Could you check a few things on this model? Use its own coordinates, in mm. A direction names the side the tool comes from. Give positions to 0.01 mm unless a question says otherwise; leave off trailing zeros. Loops run counter-clockwise (first coordinate to the right, second up) from the corner with the lowest first, then second, coordinate; pieces in that order, holes last. Notation, with made-up numbers: (15, 41) -> (60, 41) arc R9 cw to (60, 48) -> close; hole circle Ø9 at (24, -36). An arc over 180 degrees is marked (long way). Put each result on its own line as item: value.
```python
from build123d import *

# Parameters (mm, degrees)
F0_R     = 14
F1_DEPTH = 3
F2_R     = 4
F3_DEPTH = 1.25
F5_DEPTH = 11.5
F6_DEPTH = 25.4
F4_R     = 1.75
F7_DEPTH = 25.4


# Not quite as in the source:
# - a feature names something its author has since deleted; it is built from what else it names


with BuildPart() as f1:
    # F0 (on Top) → F1 (new body)
    with BuildSketch(Plane.XY):
        with Locations((-41.5364727378, -7.5015998445)):
            Circle(F0_R)
    extrude(amount=F1_DEPTH)

    # F2 (on face) → F3 (cut)
    with BuildSketch(Plane.XY.offset(3)):
        with Locations((-41.5364727378, -7.5015998445)):
            Circle(F2_R)
    extrude(amount=-F3_DEPTH, mode=Mode.SUBTRACT)

    # F4 (on face) → F5 (join)
    with BuildSketch(Plane.XY.offset(3)):
        with BuildLine():
            ThreePointArc((-46.2922708097, -1.256661386), (-49.6170112359, -0.6113276981), (-46.7751178459, -2.4536079239))
            ThreePointArc((-46.7751178459, -2.4536079239), (-46.4175303835, -1.9019950739), (-46.2922708097, -1.256661386))
        make_face()
        with BuildLine():
            ThreePointArc((-33.3423393435, -13.758620951), (-34.4205133346, -12.1594833352), (-36.3072565774, -12.5593585722))
            ThreePointArc((-36.3072565774, -12.5593585722), (-35.7141653523, -15.3577585668), (-33.3423393435, -13.758620951))
        make_face()
        with BuildLine():
            ThreePointArc((-46.0564111963, -13.9823979165), (-46.193904066, -13.3075304398), (-46.5844646585, -12.7402449527))
            ThreePointArc((-46.5844646585, -12.7402449527), (-49.3689183267, -14.6572653931), (-46.0564111963, -13.9823979165))
        make_face()
        with BuildLine():
            ThreePointArc((-33.5665342792, -1.0208017726), (-35.9664017559, 0.5667053577), (-36.4884808171, -2.2629547364))
            ThreePointArc((-36.4884808171, -2.2629547364), (-34.6166668026, -2.608308903), (-33.5665342792, -1.0208017726))
        make_face()
    extrude(amount=-F5_DEPTH)

    # F4 (on face) → F6 (cut)
    with BuildSketch(Plane.XY.offset(3)):
        with BuildLine():
            ThreePointArc((-39.7864727378, 1.9984001555), (-42.7739096049, 3.2358370225), (-41.5364727378, 0.2484001555))
            ThreePointArc((-41.5364727378, 0.2484001555), (-40.2990358707, 0.7609632884), (-39.7864727378, 1.9984001555))
        make_face()
        with BuildLine():
            ThreePointArc((-31.2864727378, -7.5015998445), (-33.0364727378, -5.7515998445), (-34.7864727378, -7.5015998445))
            ThreePointArc((-34.7864727378, -7.5015998445), (-33.0364727378, -9.2515998445), (-31.2864727378, -7.5015998445))
        make_face()
        with BuildLine():
            ThreePointArc((-39.7864727378, -17.0011998445), (-40.2990358707, -15.7637629775), (-41.5364727378, -15.2511998445))
            ThreePointArc((-41.5364727378, -15.2511998445), (-42.7739096049, -18.2386367116), (-39.7864727378, -17.0011998445))
        make_face()
    extrude(amount=-F6_DEPTH, mode=Mode.SUBTRACT)

    # F4 (on face) → F7 (cut)
    with BuildSketch(Plane.XY.offset(3)):
        with Locations((-50.0454727378, -7.5015998445)):
            Circle(F4_R)
    extrude(amount=-F7_DEPTH, mode=Mode.SUBTRACT)


solid = f1.part
```
1. If we section it at B-B (x = -32.75): List the corners of the cut face in (y, z) for me, then the cut area to 3 significant figures.
Recorded:
outline: (-18.4, 0) -> (-9.23, 0) -> (-9.23, 3) -> (-18.4, 3) -> close; (-5.78, 0) -> (3.4, 0) -> (3.4, 3) -> (-5.78, 3) -> close
area: 55.0 mm^2
2. Thinking about a two-plate mould opening in Y: for faces 4 (the face through (-35, -14, -8.5)), 5 (the face through (-28.18, -3.3, 1.48)), 6 (the face through (-42, -7, 1.75)), which applies, pulls with the +Y half, pulls with the -Y half, needs draft (parallel to the pull), parting line crosses it, or undercut?
Recorded:
face 4: needs draft
face 5: parting line crosses it
face 6: undercut
3. I need wall thicknesses on line 1 (Z direction, x = -44.75, y = -6.5); line 2 (Y direction, x = -48, z = -0.5); line 3 (Z direction, x = -37, y = -0.5). Which ranges of each line are inside material? Lowest first, please.
Recorded:
line 1: z = 0 to 1.75
line 2: y = -15.69 to -12.27, -2.98 to 0.47
line 3: z = 0 to 3
4. If we section it at C-C (x = -42.5): List the corners of the cut face in (y, z) for me.
Recorded:
outline: (-21.47, 0) -> (-18.46, 0) -> (-18.46, 3) -> (-21.47, 3) -> close; (-15.54, 0) -> (0.54, 0) -> (0.54, 3) -> (-3.62, 3) -> (-3.62, 1.75) -> (-11.38, 1.75) -> (-11.38, 3) -> (-15.54, 3) -> close; (3.46, 0) -> (6.47, 0) -> (6.47, 3) -> (3.46, 3) -> close
5. If we section it at D-D (z = 1): List the corners of the cut face in (x, y) for me, then the cut area to 3 significant figures.
Recorded:
outline: circle Ø28 at (-41.54, -7.5); hole circle Ø3.5 at (-50.05, -7.5); hole circle Ø3.5 at (-41.54, -17); hole circle Ø3.5 at (-41.54, 2); hole circle Ø3.5 at (-33.04, -7.5)
area: 577 mm^2
6. I'm going to push flat-ended pins straight in: pin 1 (4 mm diameter, centred on x = -50.05, y = -7.5, fed in from -Z); pin 2 (5 mm diameter, centred on x = -40.5, z = -1, fed in from +Y); pin 3 (7 mm diameter, centred on x = -41.54, y = -7.5, fed in from +Z); pin 4 (5 mm diameter, centred on y = -4, z = 1.5, fed in from -X). Where does each tip first touch, or does it pass through?
Recorded:
pin 1: stops at z = 0
pin 2: stops at y = 6.5
pin 3: stops at z = 1.75
pin 4: stops at x = -55.5
7. If we section it at A-A (z = -3.75): List the corners of the cut face in (x, y) for me (3 decimals).
Recorded:
outline: circle Ø3.45 at (-48.017, -1.257); circle Ø3.45 at (-47.781, -13.982); circle Ø3.45 at (-35.292, -1.021); circle Ø3.45 at (-35.067, -13.759)
8. For faces 1 (the face through (-45, -10, 3)), 2 (the face through (-42, -7, 0)), 3 (the face through (-45.533, -7.326, 2.384)), which set-ups out of +Z, -Z, +X, -X, +Y, -Y let a thin tool reach every point of the face, with its end or its side?
Recorded:
face 1: +Z, +X, -X, +Y, -Y
face 2: -Z
face 3: +Z
